The listing builds one solid part. Answer for the finished solid, in the listing's coordinates (mm). Give positions to 0.01 mm unless a question says otherwise; leave off trailing zeros. Order: outer loops, then holes, each group sorted by start corner. A loop starts at its lowest first (then second) coordinate and runs counter-clockwise, first axis right, second up. Notation, with made-up numbers: (85.25, -38) - (119.25, -38) arc R18 ccw to (119.25, -18) - close; hole circle Ø4 at (13.5, 36.25). An arc over 180 degrees is marked (long way). Answer as a JSON object with one key per item and string values. Group by question number.
Q1. A cutting plane is placed at C-C, the plane z = 0. Give the vertices of the cut face in (x, y), and give its area (3 significant figures).
Q2. Consider line 1 (Y direction, x = -4.75, z = -1.5); line 2 (Z direction, x = 3.25, y = -3.75); line 3 (X direction, y = -7.25, z = -4.5). Determine where each line is inside the solid, lowest interval first.
Q3. A cutting plane is placed at D-D, the plane x = 2. Give the vertices of the cut face in (y, z), and give its area (3 significant figures).
Q4. Given pin 1 (1.5 mm diameter, centred on x = 0, z = 2, fed in from +Y); pin 2 (5 mm diameter, centred on x = 0.5, y = 3.5, fed in from -Z), each flat-ended and moving along its own axis, determine where each tip first touches the part or whether it passes through.
Q5. A cutting plane is placed at A-A, the plane x = 0. Give the vertices of the cut face in (y, z), and give its area (3 significant figures).
Q6. A cutting plane is placed at B-B, the plane y = 4.5. Give the vertices of the cut face in (x, z), and give its area (3 significant figures).
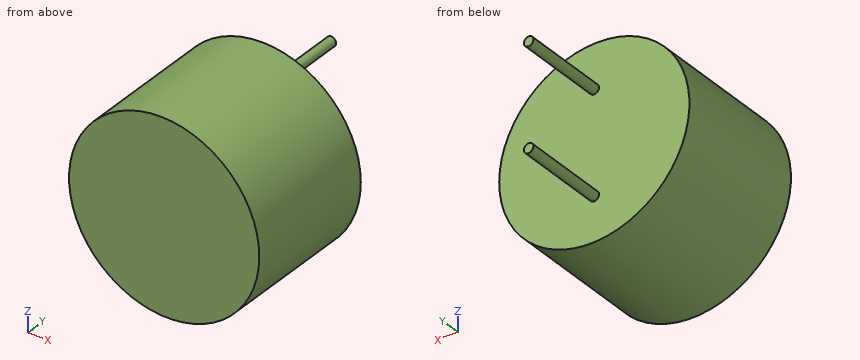
from build123d import *

# Parameters (mm, degrees)
F0_R     = 6
F1_DEPTH = 8.5
F2_R     = 0.3
F3_DEPTH = 5.5


with BuildPart() as f1:
    # F0 (on Front) → F1 (new body)
    with BuildSketch(Plane.XZ):
        Circle(F0_R)
    extrude(amount=F1_DEPTH)

    # F2 (on face) → F3 (join)
    with BuildSketch(Plane(origin=(0, 0, 0), x_dir=(-1, 0, 0), z_dir=(0, 1, 0))):
        with Locations((0, 3.22822)):
            Circle(F2_R)
        with Locations((0, -3.22822)):
            Circle(F2_R)
    extrude(amount=F3_DEPTH)


solid = f1.part
Reply:
{
 "1": {"outline": "(-6, -8.5) - (6, -8.5) - (6, 0) - (-6, 0) - close", "area": "102 mm^2"},
 "2": {"line 1": "y = -8.5 to 0", "line 2": "z = -5.04 to 5.04", "line 3": "x = -3.97 to 3.97"},
 "3": {"outline": "(-8.5, -5.66) - (0, -5.66) - (0, 5.66) - (-8.5, 5.66) - close", "area": "96.2 mm^2"},
 "4": {"pin 1": "stops at y = 0", "pin 2": "stops at z = -3.53"},
 "5": {"outline": "(-8.5, -6) - (0, -6) - (0, -3.53) - (5.5, -3.53) - (5.5, -2.93) - (0, -2.93) - (0, 2.93) - (5.5, 2.93) - (5.5, 3.53) - (0, 3.53) - (0, 6) - (-8.5, 6) - close", "area": "109 mm^2"},
 "6": {"outline": "circle Ø0.6 at (0, -3.23); circle Ø0.6 at (0, 3.23)", "area": "0.565 mm^2"}
}
